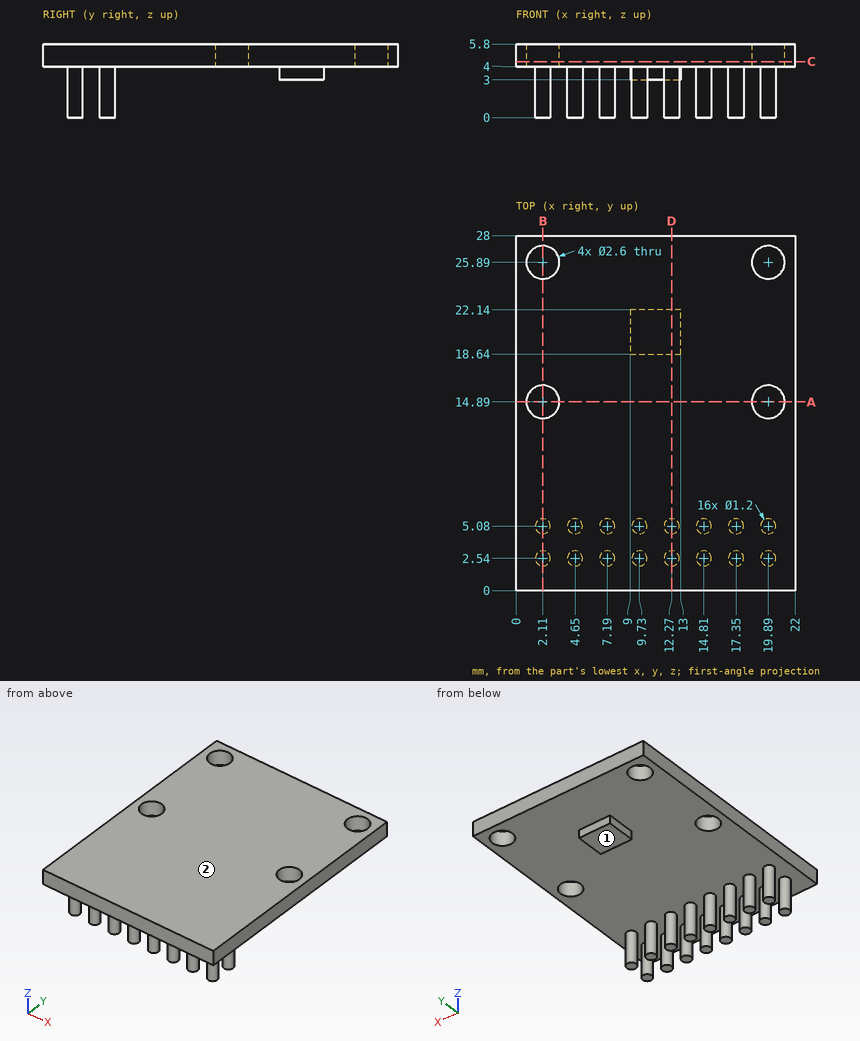
Verification items for this drawing (mm, ordinates from the low corner). A direction names the side the tool comes from. Give positions to 0.01 mm unless a question says otherwise; leave off trailing zeros. Write each loop counter-clockwise with the first axis right and the second up, starting at its lowest first coordinate (ties: lowest second). Pieces come first, ordered by that corner, then holes.
1) Section check C-C, the plane z = 4.4. Record the boundary of the cut face in (x, y).
2) Material ranges on L1, parallel to Y at x = 2.11, z = 4.4; L2, parallel to Y at x = 9.5, z = 3.75; L3, parallel to Z at x = 5.5, y = 21.5, recorded low to high.
3) Section check A-A, the plane y = 14.89. Record the boundary of the cut face in (x, z).
4) Access from +Z, -Z, +X, -X, +Y, -Y to the whole of each face (thin tool, end or side, straight path). Record for the marked faces 1 and 2.
5) Section check D-D, the plane x = 12.27. Record the boundary of the cut face in (y, z), and give its area (3 significant figures).
6) Gauge pin test, flat ends, axial feed: pin 1 (1.6 mm diameter, centred on x = 19.89, y = 25.89, fed in from +Z); pin 2 (1.5 mm diameter, centred on x = 11.5, z = 2.5, fed in from -Y); pin 3 (0.5 mm diameter, centred on y = 20.5, z = 3.5, fed in from +X); pin 4 (3 mm diameter, centred on x = 2.11, y = 14.89, fed in from -Z). Record the tip position at first contact, or that the pin passes through.
7) Section check B-B, the plane x = 2.11. Record the boundary of the cut face in (y, z).
Computed:
1. outline: (0, 0) - (22, 0) - (22, 28) - (0, 28) - close; hole circle Ø2.6 at (2.11, 14.89); hole circle Ø2.6 at (2.11, 25.89); hole circle Ø2.6 at (19.89, 14.89); hole circle Ø2.6 at (19.89, 25.89)
2. L1: y = 0 to 13.59, 16.19 to 24.59, 27.19 to 28
2. L2: y = 1.99 to 3.09, 4.53 to 5.63, 18.64 to 22.14
2. L3: z = 4 to 5.8
3. outline: (0, 4) - (0.81, 4) - (0.81, 5.8) - (0, 5.8) - close; (3.41, 4) - (18.59, 4) - (18.59, 5.8) - (3.41, 5.8) - close; (21.19, 4) - (22, 4) - (22, 5.8) - (21.19, 5.8) - close
4. face 1: -Z, +X, -X, +Y
4. face 2: +Z, +X, -X, +Y, -Y
5. outline: (0, 4) - (1.94, 4) - (1.94, 0) - (3.14, 0) - (3.14, 4) - (4.48, 4) - (4.48, 0) - (5.68, 0) - (5.68, 4) - (18.64, 4) - (18.64, 3) - (22.14, 3) - (22.14, 4) - (28, 4) - (28, 5.8) - (0, 5.8) - close
5. area: 63.5 mm2
6. pin 1: passes through
6. pin 2: stops at y = 1.94
6. pin 3: stops at x = 13
6. pin 4: stops at z = 4
7. outline: (0, 4) - (1.94, 4) - (1.94, 0) - (3.14, 0) - (3.14, 4) - (4.48, 4) - (4.48, 0) - (5.68, 0) - (5.68, 4) - (13.59, 4) - (13.59, 5.8) - (0, 5.8) - close; (16.19, 4) - (24.59, 4) - (24.59, 5.8) - (16.19, 5.8) - close; (27.19, 4) - (28, 4) - (28, 5.8) - (27.19, 5.8) - close
